from build123d import *

# Parameters (mm, degrees)
F2_R = 0.835


with BuildPart() as f3:
    # F3: sweep along a path in F0
    with BuildLine(Plane.XZ) as f3_path:
        Line((-5, 0), (-2.8, 0))
        ThreePointArc((-2.8, 0), (-2.301935, 0.150379), (-1.970312, 0.551263))
        Line((-1.970312, 0.551263), (-1.729688, 1.123737))
        ThreePointArc((-1.729688, 1.123737), (-0.722123, 1.657247), (0, 0.775))
        Line((0, 0.775), (0, 0))
        Line((0, 0), (0, -0.775))
        ThreePointArc((0, -0.775), (0.722123, -1.657247), (1.729688, -1.123737))
        Line((1.729688, -1.123737), (1.970312, -0.551263))
        ThreePointArc((1.970312, -0.551263), (2.301935, -0.150379), (2.8, 0))
        Line((2.8, 0), (5, 0))
    # F2 (on plane+point) → F3 (sweep)
    with BuildSketch(Plane.YZ.offset(-5)):
        Circle(F2_R)
    sweep(path=f3_path.line)


solid = f3.part
The listing builds one solid part. Answer for the finished solid, in the listing's coordinates (mm). A direction names the side the tool comes from. Round coordinates to 2 decimals unless told otherwise and drop trailing zeros. Loops run counter-clockwise (first coordinate to the right, second up) from the corner with the lowest first, then second, coordinate; pieces in that order, holes last. Notation, with made-up numbers: M -20.75,60 L 26.25,60 A22 cw 26.25,74 Z; hole C -13.75,12.25 d7. An arc over 180 degrees is marked long. Return JSON: item names as keys, results as strings.
Q1. Which of the six approach directions +Z, -Z, +X, -X, +Y, -Y give full straight-line access (tool end or side, diameter ignored) to faces 1 (the face through (5, 0, 0)), 2 (the face through (-3.885, -0.181, -0.815)), 3 (the face through (3.915, -0.181, -0.815))?
Results list:
{"face 1": "+Z, -Z, +X, +Y, -Y", "face 2": "-X", "face 3": "+X"}
Q2. Find section B-B, the plane x = 3. Determine the outline of the cut face in (y, z) (3 decimals), plus the area to 3 significant figures.
Results list:
{"outline": "C 0,0 d1.67", "area": "2.19 mm2"}
Q3. Find the intervals of material crossed by line 1 along X through (y, z) = (-0.1, -0.3); line 2 along X through (y, z) = (0.55, 0.4); line 3 along Z through (x, y) = (-3, -0.35), in increasing order. Write a range as from..to.
Results list:
{"line 1": "x = -5..-1.56, -0.83..0.83, 1.18..5", "line 2": "x = -5..-1.35, -0.63..0.63, 2..5", "line 3": "z = -0.76..0.76"}
Q4. Find section A-A, the plane z = 0. State how many separate pieces and enclosed holes the cut face has, plus the area to 3 significant figures.
Results list:
{"separate pieces": "3", "enclosed holes": "0", "area": "13.7 mm2"}
